Verification items for the finished model (mm, model axes). Face numbers are marked on the shaded views. A direction names the side the tool comes from. Coordinates: 2 decimals unless noted, no trailing zeros. Loops run counter-clockwise (first coordinate to the right, second up) from the corner with the lowest first, then second, coordinate; pieces in that order, holes last. Notation, with made-up numbers: (23, 39) - (37, 39) arc R19 cw to (37, 75) - close; hole circle Ø5 at (84.25, 51.5). An arc over 180 degrees is marked (long way). One line per item, written item: value. Start each with the question number.
(1) Thickness scan on probe 1 along Y at (x, z) = (69, 0.5); probe 2 along Y at (x, z) = (175, 6.5); probe 3 along X at (y, z) = (-65, 6.5). Record the ranges inside material, lowest first. Write a range as [from, to].
(2) Gauge pin test, flat ends, axial feed: P1, Ø4, axis at y = -74.5, z = 8.5, coming from the -X side; P2, Ø2.5, axis at y = -78, z = 3.5, coming from the -X side; P3, Ø1.5, axis at y = -74, z = 3, coming from the -X side. Record the tip position at first contact, or that the pin passes through.
(3) Section check B-B (x = 25). Record the boundary of the cut face in (y, z).
(4) Draft check along X on the marked faces 3, 4, 5 and 6. Enter one of: +X half, -X half, draft (parallel to the pull), parting line (faces both ways), or undercut.
(5) Section check A-A (x = 134). Record the boundary of the cut face in (y, z), plus the area to 3 significant figures.
(6) Set-up check for the marked faces 1 and 2: record each of +Z, -Z, +X, -X, +Y, -Y from which the full face is reachable in a straight line by a thin tool's end or side.
(7) Section check D-D (x = 61). Record the boundary of the cut face in (y, z).
(8) Section check C-C (y = -30). Count the separate pieces of the cut face and the enclosed holes in it, plus the area to 3 significant figures.
```python
from build123d import *

# Parameters (mm, degrees)
SKETCH_W        = 160
SKETCH_H        = 90
SKETCH_R        = 1.5625
PAD_DEPTH       = 10
POCKET_DEPTH    = 5
FILLET_R        = 20
FILLET001_R     = 30
POCKET001_DEPTH = 10.001
FILLET002_R     = 3
SKETCH003_W     = 59.09549
SKETCH003_H     = 69
POCKET002_DEPTH = 2
FILLET003_R     = 2
POCKET003_DEPTH = 2


with BuildPart() as part:
    # Sketch → Pad (new body)
    with BuildSketch(Plane.XY):
        with Locations((100, -45)):
            Rectangle(SKETCH_W, SKETCH_H)
        with Locations((175, -10)):
            Circle(SKETCH_R, mode=Mode.SUBTRACT)
        with Locations((175, -30)):
            Circle(SKETCH_R, mode=Mode.SUBTRACT)
        with Locations((25, -10)):
            Circle(SKETCH_R, mode=Mode.SUBTRACT)
        with Locations((25, -30)):
            Circle(SKETCH_R, mode=Mode.SUBTRACT)
        with BuildLine():
            ThreePointArc((95.0113, -23.9887), (92.0113, -20.9887), (89.0113, -23.9887))
            Line((89.0113, -23.9887), (89.0113, -33.9887))
            ThreePointArc((89.0113, -33.9887), (92.0113, -36.9887), (95.0113, -33.9887))
            Line((95.0113, -23.9887), (95.0113, -33.9887))
        make_face(mode=Mode.SUBTRACT)
        with BuildLine():
            ThreePointArc((88, -47.5), (68.5, -28), (49, -47.5))
            Line((49, -47.5), (49, -57.5))
            ThreePointArc((49, -57.5), (68.5, -77), (88, -57.5))
            Line((88, -47.5), (88, -57.5))
        make_face(mode=Mode.SUBTRACT)
        with BuildLine():
            ThreePointArc((95.0113, -71.0113), (92.0113, -68.0113), (89.0113, -71.0113))
            Line((89.0113, -71.0113), (89.0113, -81.0113))
            ThreePointArc((89.0113, -81.0113), (92.0113, -84.0113), (95.0113, -81.0113))
            Line((95.0113, -71.0113), (95.0113, -81.0113))
        make_face(mode=Mode.SUBTRACT)
        with BuildLine():
            ThreePointArc((47.9887, -71.0113), (44.9887, -68.0113), (41.9887, -71.0113))
            Line((41.9887, -71.0113), (41.9887, -81.0113))
            ThreePointArc((41.9887, -81.0113), (44.9887, -84.0113), (47.9887, -81.0113))
            Line((47.9887, -71.0113), (47.9887, -81.0113))
        make_face(mode=Mode.SUBTRACT)
        with BuildLine():
            ThreePointArc((47.9887, -23.9887), (44.9887, -20.9887), (41.9887, -23.9887))
            Line((41.9887, -23.9887), (41.9887, -33.9887))
            ThreePointArc((41.9887, -33.9887), (44.9887, -36.9887), (47.9887, -33.9887))
            Line((47.9887, -23.9887), (47.9887, -33.9887))
        make_face(mode=Mode.SUBTRACT)
    extrude(amount=PAD_DEPTH)

    # Sketch001 (on Face30 of Pad) → Pocket (cut)
    with BuildSketch(Plane.XY.offset(10)):
        with BuildLine():
            ThreePointArc((98.5113, -23.9887), (92.0113, -17.4887), (85.5113, -23.9887))
            Line((85.5113, -23.9887), (85.5113, -33.9887))
            ThreePointArc((85.5113, -33.9887), (92.0113, -40.4887), (98.5113, -33.9887))
            Line((98.5113, -23.9887), (98.5113, -33.9887))
        make_face()
        with BuildLine():
            ThreePointArc((51.4887, -23.9887), (44.9887, -17.4887), (38.4887, -23.9887))
            Line((38.4887, -23.9887), (38.4887, -33.9887))
            ThreePointArc((38.4887, -33.9887), (44.9887, -40.4887), (51.4887, -33.9887))
            Line((51.4887, -23.9887), (51.4887, -33.9887))
        make_face()
        with BuildLine():
            ThreePointArc((98.5113, -71.0113), (92.0113, -64.5113), (85.5113, -71.0113))
            Line((85.5113, -71.0113), (85.5113, -81.0113))
            ThreePointArc((85.5113, -81.0113), (92.0113, -87.5113), (98.5113, -81.0113))
            Line((98.5113, -71.0113), (98.5113, -81.0113))
        make_face()
        with BuildLine():
            ThreePointArc((51.4887, -71.0113), (44.9887, -64.5113), (38.4887, -71.0113))
            Line((38.4887, -71.0113), (38.4887, -81.0113))
            ThreePointArc((38.4887, -81.0113), (44.9887, -87.5113), (51.4887, -81.0113))
            Line((51.4887, -71.0113), (51.4887, -81.0113))
        make_face()
    extrude(amount=-POCKET_DEPTH, mode=Mode.SUBTRACT)

    # Fillet
    fillet_edges = [part.edges().sort_by_distance(p)[0] for p in [
        (20, -90, 5),
    ]]
    fillet(fillet_edges, radius=FILLET_R)

    # Fillet001
    fillet001_edges = [part.edges().sort_by_distance(p)[0] for p in [
        (180, -90, 5),
    ]]
    fillet(fillet001_edges, radius=FILLET001_R)

    # Sketch002 → Pocket001 (cut, through all)
    with BuildSketch(Plane.XY.offset(10)):
        with BuildLine():
            ThreePointArc((151, -38.5), (131.5, -19), (112, -38.5))
            Line((112, -38.5), (112, -58.5))
            ThreePointArc((112, -58.5), (131.5, -78), (151, -58.5))
            Line((151, -38.5), (151, -58.5))
        make_face()
    extrude(amount=-POCKET001_DEPTH, mode=Mode.SUBTRACT)

    # Fillet002
    fillet002_edges = [part.edges().sort_by_distance(p)[0] for p in [
        (20, 0, 5),
        (180, 0, 5),
    ]]
    fillet(fillet002_edges, radius=FILLET002_R)

    # Sketch003 (on Face38 of Fillet002) → Pocket002 (cut)
    with BuildSketch(Plane.XY):
        with Locations((68.547745, -52.5)):
            Rectangle(SKETCH003_W, SKETCH003_H)
    extrude(amount=POCKET002_DEPTH, mode=Mode.SUBTRACT)

    # Fillet003
    fillet003_edges = [part.edges().sort_by_distance(p)[0] for p in [
        (98.09549, -18, 1),
        (39, -18, 1),
        (39, -87, 1),
        (98.09549, -87, 1),
    ]]
    fillet(fillet003_edges, radius=FILLET003_R)

    # Sketch004 (on Face27 of Fillet003) → Pocket003 (cut)
    with BuildSketch(Plane(origin=(37, -216, 10), x_dir=(0, 1, 0), z_dir=(0, 0, 1))):
        with BuildLine():
            Line((145.517159, -116.903893), (150.632976, -116.903893))
            ThreePointArc((152.318723, -124.528938), (154.676782, -120.008753), (150.632976, -116.903893))
            ThreePointArc((150.000824, -136.237228), (156.909165, -131.521294), (152.318723, -124.528938))
            Line((150.000824, -136.237228), (145.517159, -136.237228))
            Line((145.517159, -136.237228), (145.517159, -116.903893))
        make_face()
        with BuildLine():
            Line((165.495066, -116.903893), (159.00824, -116.903893))
            Line((159.00824, -116.903893), (159.00824, -136.362732))
            Line((159.00824, -136.362732), (163.24652, -136.362732))
            Line((163.24652, -136.362732), (163.24652, -127.595039))
            Line((163.24652, -127.595039), (169.794234, -136.298567))
            Line((169.794234, -136.298567), (174.341334, -136.298567))
            Line((174.341334, -136.298567), (166.926646, -126.442617))
            ThreePointArc((166.926646, -126.442617), (170.507239, -121.02845), (165.495066, -116.903893))
        make_face()
    extrude(amount=-POCKET003_DEPTH, mode=Mode.SUBTRACT)


solid = part.part
```
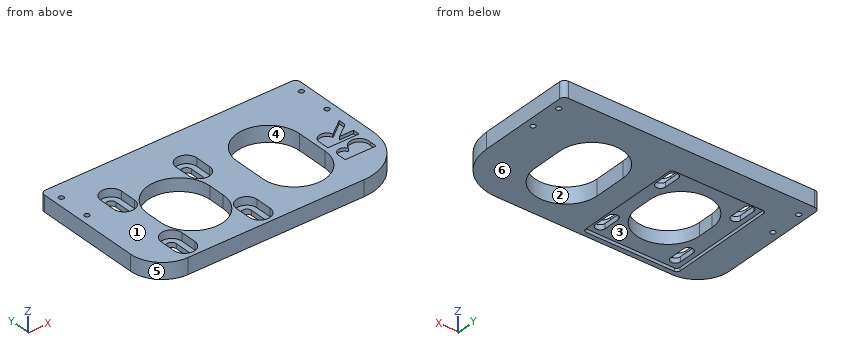
Responses:
1. probe 1: y = [-90, -87], [-18, 0]
1. probe 2: y = [-76.58, -31.56], [-28.44, -11.56], [-8.44, 0]
1. probe 3: x = [20, 42.52], [47.46, 50.5], [86.5, 89.54], [94.48, 113.12], [149.88, 179.58]
2. P1: stops at x = 20.16
2. P2: stops at x = 21.17
2. P3: stops at x = 20.27
3. outline: (-83.23, 0) - (-31.56, 0) - (-31.56, 10) - (-83.23, 10) - close; (-28.44, 0) - (-11.56, 0) - (-11.56, 10) - (-28.44, 10) - close; (-8.44, 0) - (0, 0) - (0, 10) - (-8.44, 10) - close
4. face 3: undercut
4. face 4: undercut
4. face 5: -X half
4. face 6: draft
5. outline: (-90, 0) - (-77.84, 0) - (-77.84, 10) - (-90, 10) - close; (-19.16, 0) - (0, 0) - (0, 10) - (-19.16, 10) - close
5. area: 313 mm²
6. face 1: +Z, +X, -X, +Y, -Y
6. face 2: +Z, -Z
7. outline: (-90, 0) - (-87, 0) - (-87, 2) - (-75.5, 2) - (-75.5, 10) - (-90, 10) - close; (-29.5, 2) - (-18, 2) - (-18, 0) - (0, 0) - (0, 10) - (-29.5, 10) - close
8. separate pieces: 7
8. enclosed holes: 0
8. area: 765 mm²
